The model under review builds one solid part; all positions refer to its coordinate system, in mm. A direction names the side the tool comes from. Round coordinates to 2 decimals unless told otherwise and drop trailing zeros. Loops run counter-clockwise (first coordinate to the right, second up) from the corner with the lowest first, then second, coordinate; pieces in that order, holes last. Notation, with made-up numbers: M 72.25,-3.5 L 115.25,-3.5 A25 ccw 115.25,26.5 Z; hole C 7.5,-3 d10. An arc over 180 degrees is marked long. Return JSON: item names as keys, results as strings. Group by question number.
Q1. Draft analysis for pull direction Y (two halves, no side actions). For faces 1 (the face through (-74.488, 2.972, -1.565)), 2 (the face through (-76.516, 17, -2)), 3 (the face through (-74.488, 31.028, -1.565)), 4 (the face through (-56.547, 16.421, -1.565)), state which applies: pulls with the +Y half, pulls with the -Y half, needs draft (parallel to the pull), parting line crosses it, or undercut.
Q2. To check wall thickness, follow line 1 along Y through (x, z) = (-43.81, -1.55); line 2 along X through (y, z) = (16.5, -2.95); line 3 along X through (y, z) = (21.5, -2.35). State the ranges of each line that lie inside material, in increasing order.
Q3. Consider section B-B (x = -43.81). State the section outline as (y, z) points (3 decimals), and give its area (3 significant figures).
Q4. Consider section A-A (y = 14.9). State the section outline as (x, z) points (3 decimals).
Q5. For faces 5 (the face through (19.998, 19.898, -1.565)), 6 (the face through (-23, 33, -2)), list the 3-axis set-ups (+Z, -Z, +X, -X, +Y, -Y) from which the entire face can be reached by the end or side of a thin tool; tool diameter is ignored.
Q6. Consider section D-D (x = -20). State the section outline as (y, z) points (3 decimals).
Q7. Clearance check with a flat-ended pin moving along its axis: pin 1 Ø3 at (x, y) = (-71.516, 14.9) entering from -Z. State where the tip first meets the part, or that it passes through.
Q8. Consider section C-C (z = -0.7). State the section outline as (x, y) points, and give its area (3 significant figures).
from build123d import *

# Parameters (mm, degrees)
SKETCH1_W             = 104.516
SKETCH1_H             = 32
SKETCH1_R             = 2.4
SKETCH1_R_2           = 1.8034
BOSS_EXTRUDE1_DEPTH   = 3.175
M4X0_7_TAPPED_HOLE1_D = 3.3
CHAMFER1_SIZE         = 4
F_6_32_TAPPED_HOLE1_D = 2.7051


with BuildPart() as part:
    # Sketch1 → Boss-Extrude1 (new body)
    with BuildSketch(Plane.XY):
        with Locations((-24.258, 17)):
            Rectangle(SKETCH1_W, SKETCH1_H)
        with Locations((-64.516, 25.4)):
            Circle(SKETCH1_R, mode=Mode.SUBTRACT)
        with Locations((-57.516, 14.9)):
            Circle(SKETCH1_R_2, mode=Mode.SUBTRACT)
        with Locations((-71.516, 14.9)):
            Circle(SKETCH1_R_2, mode=Mode.SUBTRACT)
        with BuildLine():
            Line((22.198129856, 27.852934279), (22.198129856, 22.147065721))
            ThreePointArc((22.198129856, 22.147065721), (19.948129856, 19.897065721), (17.698129856, 22.147065721))
            Line((17.698129856, 22.147065721), (17.698129856, 27.852934279))
            ThreePointArc((17.698129856, 27.852934279), (19.948129856, 30.102934279), (22.198129856, 27.852934279))
        make_face(mode=Mode.SUBTRACT)
    extrude(amount=-BOSS_EXTRUDE1_DEPTH)

    # M4x0.7 Tapped Hole1 (through all)
    with Locations(Plane(origin=(0, 0, -3.175), x_dir=(-1, 0, 0), z_dir=(0, 0, -1))):
        with Locations((20, 25)):
            Hole(M4X0_7_TAPPED_HOLE1_D / 2)

    # Chamfer1
    chamfer1_edges = [part.edges().sort_by_distance(p)[0] for p in [
        (-76.516, 1, -1.5875),
        (-76.516, 33, -1.5875),
    ]]
    chamfer(chamfer1_edges, length=CHAMFER1_SIZE)

    # #6-32 Tapped Hole1 (through all)
    with Locations(Plane.XY):
        with Locations((-43.81, 29.3078)):
            Hole(F_6_32_TAPPED_HOLE1_D / 2)


solid = part.part
Values:
{
 "1": {"face 1": "pulls with the -Y half", "face 2": "needs draft", "face 3": "pulls with the +Y half", "face 4": "undercut"},
 "2": {"line 1": "y = 1 to 27.96, 30.66 to 33", "line 2": "x = -76.52 to -72.35, -70.68 to -58.35, -56.68 to 28", "line 3": "x = -76.52 to 17.79, 22.1 to 28"},
 "3": {"outline": "M 1,-3.175 L 27.955,-3.175 L 27.955,0 L 1,0 Z; M 30.66,-3.175 L 33,-3.175 L 33,0 L 30.66,0 Z", "area": "93.0 mm2"},
 "4": {"outline": "M -76.516,-3.175 L -73.319,-3.175 L -73.319,0 L -76.516,0 Z; M -69.713,-3.175 L -59.319,-3.175 L -59.319,0 L -69.713,0 Z; M -55.713,-3.175 L 28,-3.175 L 28,0 L -55.713,0 Z"},
 "5": {"face 5": "+Z, -Z", "face 6": "+Z, -Z, +X, -X, +Y"},
 "6": {"outline": "M 1,-3.175 L 23.35,-3.175 L 23.35,0 L 1,0 Z; M 26.65,-3.175 L 33,-3.175 L 33,0 L 26.65,0 Z"},
 "7": {"pin 1": "passes through"},
 "8": {"outline": "M -76.52,5 L -72.52,1 L 28,1 L 28,33 L -72.52,33 L -76.52,29 Z; hole C -71.52,14.9 d3.61; hole C -64.52,25.4 d4.8; hole C -57.52,14.9 d3.61; hole C -43.81,29.31 d2.71; hole C -20,25 d3.3; hole M 17.7,22.15 A2.25 ccw 22.2,22.15 L 22.2,27.85 A2.25 ccw 17.7,27.85 Z", "area": "3,230 mm2"}
}
